Can you work these out from the model? Positions are in its coordinate system, mm. Give positions to 0.01 mm unless a question says otherwise; leave off trailing zeros. Write each loop counter-clockwise with the first axis right and the second up, starting at its lowest first coordinate (ties: lowest second). Pieces come first, ordered by that corner, then holes.
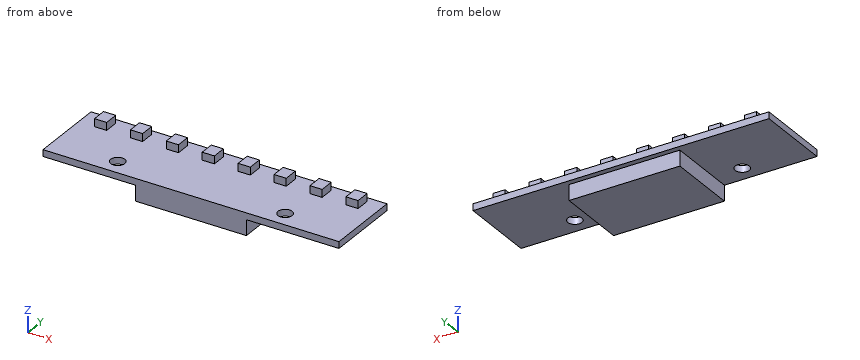
from build123d import *

# Parameters (mm, degrees)
SKETCH1_W           = 66.75
SKETCH1_H           = 17.25
BOSS_EXTRUDE1_DEPTH = 1.5
SKETCH2_W           = 2.75
SKETCH2_H           = 3.25
BOSS_EXTRUDE2_DEPTH = 1.75
LPATTERN1_COUNT     = 8
LPATTERN1_PITCH     = 8.1
SKETCH3_R           = 1.6
CUT_EXTRUDE1_DEPTH  = 2.5
SKETCH4_W           = 25
SKETCH4_H           = 16
BOSS_EXTRUDE3_DEPTH = 3.5


with BuildPart() as part:
    # Sketch1 → Boss-Extrude1 (new body)
    with BuildSketch(Plane.XY):
        with Locations((33.375, 8.625)):
            Rectangle(SKETCH1_W, SKETCH1_H)
    extrude(amount=BOSS_EXTRUDE1_DEPTH)

    # Sketch2 → Boss-Extrude2 (add)
    with BuildSketch(Plane.XY.offset(1.5)):
        with Locations((4.975, 14.375)):
            Rectangle(SKETCH2_W, SKETCH2_H)
    boss_extrude2 = extrude(amount=BOSS_EXTRUDE2_DEPTH)

    # LPattern1: Boss-Extrude2 ×8
    with Locations(*[(i * LPATTERN1_PITCH, 0, 0) for i in range(1, LPATTERN1_COUNT)]):
        add(boss_extrude2)

    # Sketch3 → Cut-Extrude1 (cut, through all)
    with BuildSketch(Plane.XY.offset(1.5)):
        with Locations((14.5, 3.75)):
            Circle(SKETCH3_R)
    cut_extrude1 = extrude(amount=-CUT_EXTRUDE1_DEPTH, mode=Mode.SUBTRACT)

    # Mirror1: Cut-Extrude1 across plane
    add(cut_extrude1.mirror(Plane.ZY.offset(-33.375)), mode=Mode.SUBTRACT)

    # Sketch4 → Boss-Extrude3 (add)
    with BuildSketch(Plane(origin=(0, 0, 0), x_dir=(-1, 0, 0), z_dir=(0, 0, -1))):
        with Locations((-33.375, 8)):
            Rectangle(SKETCH4_W, SKETCH4_H)
    extrude(amount=BOSS_EXTRUDE3_DEPTH)


solid = part.part
(1) Will these pins go through, and if not, where does the flat tip stop? P1, Ø1.9, axis at y = 13.5, z = 2.5, coming from the +X side; P2, Ø0.9, axis at x = 21, z = 2.5, coming from the -Y side; P3, Ø1.4, axis at x = 53.5, z = 2.5, coming from the +Y side; P4, Ø1.9, axis at x = 14.5, y = 3.75, coming from the -Z side.
Returned:
P1: stops at x = 63.05
P2: stops at y = 12.75
P3: stops at y = 16
P4: passes through
(2) Imagine slicing it at D-D, the plane z = -1.5. Write out the boundary of the cut face in (x, y) (3 decimals), plus the area to 3 significant figures.
Returned:
outline: (20.875, 0) - (45.875, 0) - (45.875, 16) - (20.875, 16) - close
area: 400 mm2
(3) Imagine slicing it at C-C, the plane x = 47.5. Write out the boundary of the cut face in (y, z).
Returned:
outline: (0, 0) - (17.25, 0) - (17.25, 1.5) - (0, 1.5) - close
(4) Imagine slicing it at B-B, the plane y = 9. Write out the boundary of the cut face in (x, z) (3 decimals), plus the area to 3 significant figures.
Returned:
outline: (0, 0) - (20.875, 0) - (20.875, -3.5) - (45.875, -3.5) - (45.875, 0) - (66.75, 0) - (66.75, 1.5) - (0, 1.5) - close
area: 188 mm2
(5) Imagine slicing it at A-A, the plane y = 3.75. Write out the boundary of the cut face in (x, z) (3 decimals).
Returned:
outline: (0, 0) - (12.9, 0) - (12.9, 1.5) - (0, 1.5) - close; (16.1, 0) - (20.875, 0) - (20.875, -3.5) - (45.875, -3.5) - (45.875, 0) - (50.65, 0) - (50.65, 1.5) - (16.1, 1.5) - close; (53.85, 0) - (66.75, 0) - (66.75, 1.5) - (53.85, 1.5) - close
(6) If I drill on L1, parallel to Y at x = 52.25, z = 0.7; L2, parallel to Z at x = 31.5, y = 8.25; L3, parallel to Y at x = 38, z = -2, over which ranges is the centre line in solid material (lowest first)?
Returned:
L1: y = 0 to 2.15, 5.35 to 17.25
L2: z = -3.5 to 1.5
L3: y = 0 to 16
